from build123d import *

# Parameters (mm, degrees)
SKETCH_1_W          = 45
SKETCH_1_H          = 1.8
EXTRUDE_1_DEPTH     = 18
SKETCH_2_W          = 15
SKETCH_2_H          = 15
CUT_EXTRUDE_1_DEPTH = 15
EXTRUDE_2_DEPTH     = 45
CUT_EXTRUDE_2_DEPTH = 45
CUT_EXTRUDE_3_DEPTH = 45
FILLET_1_R          = 2
FILLET_2_R          = 2


with BuildPart() as part:
    # 草图1 → 凸台-拉伸1 (new body)
    with BuildSketch(Plane(origin=(0, 0, 0), x_dir=(0, 0, -1), z_dir=(1, 0, 0))):
        Rectangle(SKETCH_1_W, SKETCH_1_H)
    extrude(amount=EXTRUDE_1_DEPTH)

    # 草图2 → 切除-拉伸1 (cut)
    with BuildSketch(Plane(origin=(0, 0.9, 0), x_dir=(1, 0, 0), z_dir=(0, 1, 0))):
        with Locations((7.5, 0)):
            Rectangle(SKETCH_2_W, SKETCH_2_H)
    extrude(amount=-CUT_EXTRUDE_1_DEPTH, mode=Mode.SUBTRACT)

    # 草图4 → 凸台-拉伸2 (add)
    with BuildSketch(Plane(origin=(0, 0, -22.5), x_dir=(-1, 0, 0), z_dir=(0, 0, -1))):
        Polygon((-18, -0.9), (-102.602540378, -49.745299462), (-104.602540378, -46.281197846), (-22.882308546, 0.9), (-18, 0.9), align=None)
    extrude(amount=-EXTRUDE_2_DEPTH)

    # 草图5 → 切除-拉伸2 (cut)
    with BuildSketch(Plane.XY.offset(22.5)):
        Polygon((102.602540378, -45.126497308), (102.602540378, -49.745299462), (104.602540378, -46.281197846), align=None)
    extrude(amount=-CUT_EXTRUDE_2_DEPTH, mode=Mode.SUBTRACT)

    # 草图6 → 切除-拉伸3 (cut)
    with BuildSketch(Plane.XY.offset(22.5)):
        Polygon((102.602540378, -45.126497308), (102.349506488, -45.287661356), (102.602540378, -45.448825404), align=None)
        Polygon((102.602540378, -45.476497308), (102.349506488, -45.637661356), (102.602540378, -45.798825404), align=None)
        Polygon((102.602540378, -45.826497308), (102.349506488, -45.987661356), (102.602540378, -46.148825404), align=None)
        Polygon((102.602540378, -46.176497308), (102.349506488, -46.337661356), (102.602540378, -46.498825404), align=None)
        Polygon((102.602540378, -46.526497308), (102.349506488, -46.687661356), (102.602540378, -46.848825404), align=None)
        Polygon((102.602540378, -46.876497308), (102.349506488, -47.037661356), (102.602540378, -47.198825404), align=None)
        Polygon((102.602540378, -47.226497308), (102.349506488, -47.387661356), (102.602540378, -47.548825404), align=None)
        Polygon((102.602540378, -47.576497308), (102.349506488, -47.737661356), (102.602540378, -47.898825404), align=None)
        Polygon((102.602540378, -47.926497308), (102.349506488, -48.087661356), (102.602540378, -48.248825404), align=None)
        Polygon((102.602540378, -48.276497308), (102.349506488, -48.437661356), (102.602540378, -48.598825404), align=None)
        Polygon((102.602540378, -48.626497308), (102.349506488, -48.787661356), (102.602540378, -48.948825404), align=None)
        Polygon((102.602540378, -48.976497308), (102.349506488, -49.137661356), (102.602540378, -49.298825404), align=None)
    extrude(amount=-CUT_EXTRUDE_3_DEPTH, mode=Mode.SUBTRACT)

    # 圆角1
    fillet_1_edges = [part.edges().sort_by_distance(p)[0] for p in [
        (22.882308546, 0.9, 0),
    ]]
    fillet(fillet_1_edges, radius=FILLET_1_R)

    # 圆角2
    fillet_2_edges = [part.edges().sort_by_distance(p)[0] for p in [
        (18, -0.9, 0),
    ]]
    fillet(fillet_2_edges, radius=FILLET_2_R)


solid = part.part
Part model, mm, in its own coordinate system. A direction names the side the tool comes from. Give positions to 0.01 mm unless a question says otherwise; leave off trailing zeros. Write each loop counter-clockwise with the first axis right and the second up, starting at its lowest first coordinate (ties: lowest second). Pieces come first, ordered by that corner, then holes.
1) Cut at B-B on y = -26.5. Write the cut outline in (x, z).
Resolved:
outline: (62.34, -22.5) - (70.34, -22.5) - (70.34, 22.5) - (62.34, 22.5) - close
2) Pin check, flat tips, straight feed: pin 1 (5 mm diameter, centred on x = 9.5, z = 6, fed in from -Y); pin 2 (0.9 mm diameter, centred on y = 0.5, z = -3.5, fed in from -X); pin 3 (10 mm diameter, centred on x = 18.5, z = 17.5, fed in from -Y). Stop position of each tip, or through.
Resolved:
pin 1: stops at y = -0.9
pin 2: stops at x = 15
pin 3: stops at y = -4.08
3) Cut at A-A on x = 8. Write the cut outline in (y, z).
Resolved:
outline: (-0.9, -22.5) - (0.9, -22.5) - (0.9, -7.5) - (-0.9, -7.5) - close; (-0.9, 7.5) - (0.9, 7.5) - (0.9, 22.5) - (-0.9, 22.5) - close
4) Which spindle directions (+Z, -Z, +X, -X, +Y, -Y) get a long thin tool onto all of the face, cutting with end or side? Do faces 1 (the face through (16, -0.9, 0)), 2 (the face through (16, 0.9, 0)). Say none if no direction does.
Resolved:
face 1: +Z, -Z, -X, -Y
face 2: +Z, -Z, +X, -X, +Y
5) Cut at C-C on x = 61.5. Write the cut outline in (y, z).
Resolved:
outline: (-26.01, -22.5) - (-21.4, -22.5) - (-21.4, 22.5) - (-26.01, 22.5) - close
6) Probe L1, parallel to Y at x = 13, z = -19; L2, parallel to X at y = -34.5, z = -11; L3, parallel to X at y = -47, z = 0.5. List the from-to ranges inside material, lowest first.
Resolved:
L1: y = -0.9 to 0.9
L2: x = 76.2 to 84.2
L3: x = 97.85 to 102.41
